The listing builds one solid part. Answer for the finished solid, in the listing's coordinates (mm). A direction names the side the tool comes from. Coordinates: 2 decimals unless noted, no trailing zeros. Order: outer loops, then holes, each group sorted by start corner. A loop starts at its lowest first (then second) coordinate and runs counter-clockwise, first axis right, second up. Notation, with made-up numbers: (14.5, 77.25) -> (49.5, 77.25) arc R16 cw to (49.5, 96.25) -> close; hole circle Ø6 at (-6, -12). An arc over 180 degrees is marked (long way). Return JSON: item names as keys, results as strings.
```python
from build123d import *

# Parameters (mm, degrees)
SKETCH2_W             = 17.554431489
SKETCH2_H             = 1.95
BOSS_EXTRUDE1_DEPTH   = 8.75
BOSS_EXTRUDE1_2_DEPTH = 8.75
CUT_EXTRUDE1_DEPTH    = 26.518349076
SKETCH4_W             = 22.027215745
SKETCH4_H             = 12.505427167
BOSS_EXTRUDE2_DEPTH   = 32
SKETCH5_R             = 1.5
CUT_EXTRUDE2_DEPTH    = 12
SKETCH6_W             = 22.027215745
SKETCH6_H             = 12.505427167
SKETCH6_W_2           = 17.554431489
SKETCH6_H_2           = 1.95
CUT_EXTRUDE3_DEPTH    = 2.5
SKETCH7_R             = 1.5
CUT_EXTRUDE4_DEPTH    = 13
SKETCH8_R             = 1.5
CUT_EXTRUDE5_DEPTH    = 28
FILLET3_R             = 1
SKETCH9_W             = 22.02721574
SKETCH9_H             = 2
CUT_EXTRUDE6_DEPTH    = 11


with BuildPart() as part:
    # Sketch2 → Boss-Extrude1 (new body)
    with BuildSketch(Plane.XY):
        with Locations((-13.228930986, -27.845183414)):
            Rectangle(SKETCH2_W, SKETCH2_H)
    extrude(amount=BOSS_EXTRUDE1_DEPTH)


with BuildPart() as body_2:
    # Sketch2 → Boss-Extrude1 2 (new body)
    with BuildSketch(Plane.XY):
        with Locations((-13.228930986, -20.289756247)):
            Rectangle(SKETCH2_W, SKETCH2_H)
    extrude(amount=BOSS_EXTRUDE1_2_DEPTH)


with BuildPart() as cut_extrude1_tool:
    # Sketch3 → Cut-Extrude1 (new, through all)
    with BuildSketch(Plane(origin=(0, -19.314756247, 0), x_dir=(1, 0, 0), z_dir=(0, 1, 0))):
        with BuildLine():
            ThreePointArc((-13.228930986, -8.75), (-7.041746651, -6.187184335), (-4.478930986, 0))
            add(Edge.make_bspline(
                [(-4.478930986, 0), (1.138349918, -4.151657709), (-4.451715242, -8.75)],
                knots=[0, 0, 0, 1, 1, 1], degree=2))
            add(Edge.make_bspline(
                [(-22.006146731, -8.75), (-13.228930986, -12.473510392), (-4.451715242, -8.75)],
                knots=[0, 0, 0, 1, 1, 1], degree=2))
            add(Edge.make_bspline(
                [(-21.978930986, 0), (-25.926969228, -4.242865138), (-22.006146731, -8.75)],
                knots=[0, 0, 0, 1, 1, 1], degree=2))
            ThreePointArc((-21.978930986, 0), (-19.416115322, -6.187184335), (-13.228930986, -8.75))
        make_face()
    extrude(amount=-CUT_EXTRUDE1_DEPTH)


with BuildPart() as part_1:
    add(part.part)

    # Cut-Extrude1: cut by cut_extrude1_tool
    add(cut_extrude1_tool.part, mode=Mode.SUBTRACT)



with BuildPart() as body_2_1:
    add(body_2.part)

    # Cut-Extrude1: cut by cut_extrude1_tool
    add(cut_extrude1_tool.part, mode=Mode.SUBTRACT)


with BuildPart() as part_2:
    add(part_1.part)

    add(body_2_1.part)  # Boss-Extrude2 merges body 2
    # Sketch4 → Boss-Extrude2 (add)
    with BuildSketch(Plane(origin=(0, 0, 0), x_dir=(-1, 0, 0), z_dir=(0, 0, -1))):
        with Locations((13.242538859, -24.067469831)):
            Rectangle(SKETCH4_W, SKETCH4_H)
    extrude(amount=BOSS_EXTRUDE2_DEPTH)

    # Sketch5 → Cut-Extrude2 (cut)
    with BuildSketch(Plane(origin=(0, -19.314756247, 0), x_dir=(1, 0, 0), z_dir=(0, 1, 0))):
        with Locations(Location((-13.228930986, -2.25, 0), (0, 0, 270))):
            Circle(SKETCH5_R)
    extrude(amount=-CUT_EXTRUDE2_DEPTH, mode=Mode.SUBTRACT)

    # Sketch6 → Cut-Extrude3 (cut)
    with BuildSketch(Plane.XY):
        with Locations((-13.242538859, -24.067469831)):
            Rectangle(SKETCH6_W, SKETCH6_H)
        with Locations((-13.228930986, -27.845183414)):
            Rectangle(SKETCH6_W_2, SKETCH6_H_2, mode=Mode.SUBTRACT)
        with Locations((-13.228930986, -20.289756247)):
            Rectangle(SKETCH6_W_2, SKETCH6_H_2, mode=Mode.SUBTRACT)
    extrude(amount=-CUT_EXTRUDE3_DEPTH, mode=Mode.SUBTRACT)

    # Sketch7 → Cut-Extrude4 (cut)
    with BuildSketch(Plane(origin=(0, -17.814756247, 0), x_dir=(1, 0, 0), z_dir=(0, 1, 0))):
        with Locations(Location((-13.242538859, 25.5, 0), (0, 0, 270))):
            Circle(SKETCH7_R)
        with BuildLine():
            Line((-24.086865874, 21.155672985), (-24.256146731, 21.155672985))
            add(Edge.make_bspline(
                [(-2.228930986, 21.155672985), (11.471530889, 27.189710441), (-11.765166974, 53.431279988), (-37.007876173, 21.523583672), (-24.256146731, 21.155672985)],
                knots=[0, 0, 0, 0, 0.52011282, 1, 1, 1, 1], degree=3))
            add(Edge.make_bspline(
                [(-4.552660132, 30.311399113), (-2.685211009, 25.928521854), (-2.228930986, 21.155672985)],
                knots=[0, 0, 0, 1, 1, 1], degree=2))
            Line((-4.552660132, 30.311399113), (-13.242538859, 32))
            ThreePointArc((-13.242538859, 32), (-20.910636028, 28.823770155), (-24.086865874, 21.155672985))
        make_face()
    extrude(amount=-CUT_EXTRUDE4_DEPTH, mode=Mode.SUBTRACT)

    # Sketch8 → Cut-Extrude5 (cut)
    with BuildSketch(Plane.XY.offset(-2.5)):
        with Locations((-18.011106811, -24.06746983)):
            Circle(SKETCH8_R)
        with Locations((-8.473970906, -24.06746983)):
            Circle(SKETCH8_R)
    extrude(amount=-CUT_EXTRUDE5_DEPTH, mode=Mode.SUBTRACT)

    # Fillet3
    # the kernel refuses this fillet: 1 mm, written as the material it takes off along each edge
    with BuildSketch(Plane(origin=(-24.256146731, -15.314756247, -2.5), x_dir=(0, 0, -1), z_dir=(0, -1, 0)), Plane(origin=(-2.228930986, -32.820183414, -2.5), x_dir=(0, 0, -1), z_dir=(0, 1, 0))) as fillet3_piece_1:
        with BuildLine():
            CenterArc((FILLET3_R, FILLET3_R), FILLET3_R, 180, 90)
            Line((0, FILLET3_R), (-FILLET3_R * 0.02, FILLET3_R))
            Line((-FILLET3_R * 0.02, FILLET3_R), (-FILLET3_R * 0.02, -FILLET3_R * 0.02))
            Line((-FILLET3_R * 0.02, -FILLET3_R * 0.02), (FILLET3_R, -FILLET3_R * 0.02))
            Line((FILLET3_R, -FILLET3_R * 0.02), (FILLET3_R, 0))
        make_face()
    extrude(amount=17.505427167, mode=Mode.SUBTRACT)
    with BuildSketch(Plane(origin=(-24.256146731, -16.423026869, -21.155672985), x_dir=(1.0, 0, 2.5394386720559264e-12), z_dir=(0, -1, 0))) as fillet3_piece_2:
        with BuildLine():
            CenterArc((1, 0.556691751), FILLET3_R, 180, 33.827317624)
            Line((0, 0.556691751), (-0.02, 0.556691751))
            Line((-0.02, 0.556691751), (-0.02, 0))
            Line((-0.02, 0), (0, -0.02))
            ThreePointArc((0, -0.02), (0.084640429, -0.02), (0.152666474, -0.011133835))
            Line((0.152666474, -0.011133835), (0.169280857, 0))
        make_face()
    extrude(amount=15.288885922, mode=Mode.SUBTRACT)
    with BuildSketch(Plane(origin=(-4.552660132, -16.451585564, -30.311399113), x_dir=(0.3839298520349852, 0, 0.9233622629912891), z_dir=(0, -1, 0))) as fillet3_piece_3:
        with BuildLine():
            CenterArc((0.536514164, 0.999961682), FILLET3_R, 213.573886674, 56.927693277)
            Line((-0.296659206, 0.446949805), (-0.313322674, 0.435889568))
            Line((-0.313322674, 0.435889568), (-0.016663467, -0.011060238))
            Line((-0.016663467, -0.011060238), (-0.0001747, -0.019999237))
            ThreePointArc((-0.0001747, -0.019999237), (0.272634035, -0.021192075), (0.545443356, -0.019999234))
            Line((0.545443356, -0.019999234), (0.545268273, 0))
        make_face()
    extrude(amount=15.231768533, mode=Mode.SUBTRACT)

    # Sketch9 → Cut-Extrude6 (cut)
    with BuildSketch(Plane.XY.offset(-32.5)):
        with Locations((-13.24253886, -20.31475625)):
            Rectangle(SKETCH9_W, SKETCH9_H)
        with Locations((-13.24253886, -27.836055834)):
            Rectangle(SKETCH9_W, SKETCH9_H)
    extrude(amount=CUT_EXTRUDE6_DEPTH, mode=Mode.SUBTRACT)


solid = part_2.part
```
Item 1: The part is cut by section D-D on z = -28. Count the separate pieces of the cut face and the enclosed holes in it, plus the area to 3 significant figures.
Answer list:
{"separate pieces": "3", "enclosed holes": "2", "area": "139 mm2"}
Item 2: The part is cut by section A-A on z = 2.25. Determine the outline of the cut face in (x, y).
Answer list:
{"outline": "(-21.68, -28.82) -> (-14.73, -28.82) -> (-14.73, -26.87) -> (-21.68, -26.87) -> close; (-21.68, -21.26) -> (-14.73, -21.26) -> (-14.73, -19.31) -> (-21.68, -19.31) -> close; (-11.73, -28.82) -> (-4.77, -28.82) -> (-4.77, -26.87) -> (-11.73, -26.87) -> close; (-11.73, -21.26) -> (-4.77, -21.26) -> (-4.77, -19.31) -> (-11.73, -19.31) -> close"}
Item 3: Which of the six approach directions +Z, -Z, +X, -X, +Y, -Y give full straight-line access (tool end or side, diameter ignored) to faces 1 (the cylindrical face through (-7.043, -23.617, -16.304)), 2 (the cylindrical face through (-2.53, -24.155, -2.785)), 3 (the flat face through (-13, -28.836, -28)), 4 (the cylindrical face through (-13.2, -29.6, -27)), 5 (the flat face through (-15, -21.265, 2))?
Answer list:
{"face 1": "+Z", "face 2": "+Z, +X, +Y, -Y", "face 3": "-Z, +X, -X", "face 4": "+Y, -Y", "face 5": "+Z, +X, -X"}
Item 4: Find the intervals of material crossed by probe 1 along Y at (x, z) = (-9.75, 3); probe 2 along Y at (x, z) = (-8.5, -26); probe 3 along X at (y, z) = (-23.5, -3.5), in increasing order.
Answer list:
{"probe 1": "-28.82 to -26.87, -21.26 to -19.31", "probe 2": "-30.32 to -28.84, -26.84 to -25.57, -22.57 to -21.31, -19.31 to -17.81", "probe 3": "-24.26 to -19.4, -16.62 to -9.86, -7.09 to -2.23"}
Item 5: The part is cut by section C-C on z = -9. Determine the outline of the cut face in (x, y).
Answer list:
{"outline": "(-24.26, -30.32) -> (-2.23, -30.32) -> (-2.23, -17.81) -> (-24.26, -17.81) -> close; hole circle Ø3 at (-18.01, -24.07); hole circle Ø3 at (-8.47, -24.07)"}
Item 6: The part is cut by section B-B on x = -15.5. Determine the outline of the cut face in (y, z), plus the area to 3 significant figures.
Answer list:
{"outline": "(-30.32, -31.76) -> (-28.84, -31.76) -> (-28.84, -21.5) -> (-26.84, -21.5) -> (-26.84, -31.76) -> (-21.31, -31.76) -> (-21.31, -21.5) -> (-19.31, -21.5) -> (-19.31, -31.76) -> (-17.81, -31.76) -> (-17.81, -2.5) -> (-19.31, -2.5) -> (-19.31, 8.45) -> (-21.26, 8.45) -> (-21.26, -2.5) -> (-26.87, -2.5) -> (-26.87, 8.45) -> (-28.82, 8.45) -> (-28.82, -2.5) -> (-30.32, -2.5) -> close", "area": "368 mm2"}
Item 7: Flat-ended cylindrical pins translate along their axes: pin 1 (12.5 mm diameter, centred on x = -11, z = 5.5, fed in from +Y); pin 2 (5 mm diameter, centred on x = -13.23, z = 2.25, fed in from -Y); pin 3 (0.6 mm diameter, centred on y = -27.5, z = -1.5, fed in from +X). Find the tip coordinate at first contact, or state that the pin passes through.
Answer list:
{"pin 1": "y = -19.31", "pin 2": "y = -28.82", "pin 3": "x = -4.45"}
Item 8: Determine the mould class of faces 6 (the flat face through (-9.104, -24.037, -31.196)), 7 (the flat face through (-15, -28.82, 2)), 8 (the flat face through (-13, -24, -2.5)), 9 (the flat face through (-18, -24, -30.5)) for opening direction Y: pulls with the +Y half, pulls with the -Y half, needs draft (parallel to the pull), parting line crosses it, or undercut.
Answer list:
{"face 6": "needs draft", "face 7": "pulls with the -Y half", "face 8": "undercut", "face 9": "undercut"}
